```python
from build123d import *

# Parameters (mm, degrees)
SKETCH1_R            = 2.75
BOSS_EXTRUDE1_DEPTH  = 3
M3_CLEARANCE_HOLE1_D = 3.4
FILLET2_R            = 10


with BuildPart() as part:
    # Sketch1 → Boss-Extrude1 (new, symmetric)
    with BuildSketch(Plane(origin=(0, 0, 0), x_dir=(1, 0, 0), z_dir=(0, 1, 0))):
        with BuildLine():
            Line((-58.614111744, 67.959966353), (-53.914904373, 62.511483636))
            ThreePointArc((-53.914904373, 62.511483636), (-82.55, 0), (-53.914904373, -62.511483636))
            Line((-53.914904373, -62.511483636), (-58.614111744, -67.959966353))
            ThreePointArc((-58.614111744, -67.959966353), (-60.384815089, -73.721869234), (-57.34308106, -78.925980035))
            ThreePointArc((-57.34308106, -78.925980035), (-42.766558206, -87.684438581), (-26.890595122, -93.77864983))
            ThreePointArc((-26.890595122, -93.77864983), (-20.917021387, -92.971598421), (-17.46673379, -88.028883515))
            Line((-17.46673379, -88.028883515), (-16.066391761, -80.971436666))
            ThreePointArc((-16.066391761, -80.971436666), (0, -82.55), (16.066391761, -80.971436666))
            Line((16.066391761, -80.971436666), (17.46673379, -88.028883515))
            ThreePointArc((17.46673379, -88.028883515), (20.917021387, -92.971598421), (26.890595122, -93.77864983))
            ThreePointArc((26.890595122, -93.77864983), (42.766558206, -87.684438581), (57.34308106, -78.925980035))
            ThreePointArc((57.34308106, -78.925980035), (60.384815089, -73.721869234), (58.614111744, -67.959966353))
            Line((58.614111744, -67.959966353), (53.914904373, -62.511483636))
            ThreePointArc((53.914904373, -62.511483636), (82.55, 0), (53.914904373, 62.511483636))
            Line((53.914904373, 62.511483636), (58.614111744, 67.959966353))
            ThreePointArc((58.614111744, 67.959966353), (60.384815089, 73.721869234), (57.34308106, 78.925980035))
            ThreePointArc((57.34308106, 78.925980035), (42.766558206, 87.684438581), (26.890595122, 93.77864983))
            ThreePointArc((26.890595122, 93.77864983), (20.917021387, 92.971598421), (17.46673379, 88.028883515))
            Line((17.46673379, 88.028883515), (16.066391761, 80.971436666))
            ThreePointArc((16.066391761, 80.971436666), (0, 82.55), (-16.066391761, 80.971436666))
            Line((-16.066391761, 80.971436666), (-17.46673379, 88.028883515))
            ThreePointArc((-17.46673379, 88.028883515), (-20.917021387, 92.971598421), (-26.890595122, 93.77864983))
            ThreePointArc((-26.890595122, 93.77864983), (-42.766558206, 87.684438581), (-57.34308106, 78.925980035))
            ThreePointArc((-57.34308106, 78.925980035), (-60.384815089, 73.721869234), (-58.614111744, 67.959966353))
        make_face()
        with Locations(Location((52.934691668, -72.858352577, 0), (0, 0, 270))):
            Circle(SKETCH1_R, mode=Mode.SUBTRACT)
        with Locations(Location((52.934691668, 72.858352577, 0), (0, 0, 90))):
            Circle(SKETCH1_R, mode=Mode.SUBTRACT)
    extrude(amount=BOSS_EXTRUDE1_DEPTH, both=True)

    # M3 Clearance Hole1 (through all)
    with Locations(Plane(origin=(0, 3, 0), x_dir=(1, 0, 0), z_dir=(0, 1, 0))):
        with Locations((0, 79.5), (46.728927557, 64.316851053), (75.608993045, 24.566851053), (75.608993045, -24.566851053), (46.728927557, -64.316851053), (0, -79.5), (-46.728927557, -64.316851053), (-75.608993045, -24.566851053), (-75.608993045, 24.566851053), (-46.728927557, 64.316851053)):
            Hole(M3_CLEARANCE_HOLE1_D / 2)

    # Fillet2
    fillet2_edges = [part.edges().sort_by_distance(p)[0] for p in [
        (-53.914904373, 0, 62.511483636),
        (-53.914904373, 0, -62.511483636),
        (-16.066391761, 0, 80.971436666),
        (53.914904373, 0, 62.511483636),
        (53.914904373, 0, -62.511483636),
        (16.066391761, 0, -80.971436666),
        (-16.066391761, 0, -80.971436666),
    ]]
    fillet(fillet2_edges, radius=FILLET2_R)


solid = part.part
```
Source: CAD feature listing. Evaluate the final solid. Frame: model axes, mm. Give positions to 0.01 mm unless a question says otherwise; leave off trailing zeros. Write each loop counter-clockwise with the first axis right and the second up, starting at its lowest first coordinate (ties: lowest second). Pieces come first, ordered by that corner, then holes.
1. Section query C-C (x = -40). Return the cut outline in (y, z), then the cut area to 3 significant figures.
2. Section query A-A (y = 1). Count the separate pieces of the cut face and the enclosed holes in it, then the cut area to 3 significant figures.
3. First-contact query: pin 1 (3 mm diameter, centred on y = 1.5, z = -66, fed in from +X); pin 2 (3 mm diameter, centred on x = 11, y = 2, fed in from -Z). Flat tips, straight axial feed; report the tip coordinate or a pass-through.
4. Pull-direction query (X, two-part tool) for faces 1 (the face through (0.1, 0.04, -82.55)), 2 (the face through (-42.98, 0.04, 87.58)), 3 (the face through (-1, -3, -1)); classes: +X half, -X half, draft (parallel to the pull), parting line (faces both ways), or undercut.
5. Section query B-B (z = -32). Return the cut outline in (x, y), then the cut area to 3 significant figures.
6. Material intervals for line 1 along Z through (x, y) = (0, -0.5); line 2 along Z through (x, y) = (-74.5, -2.25); line 3 along X through (y, z) = (1, 63.5), sorted ascending.
Output values:
1. outline: (-3, -88.98) - (3, -88.98) - (3, 88.98) - (-3, 88.98) - close
1. area: 1,070 mm2
2. separate pieces: 1
2. enclosed holes: 12
2. area: 24,100 mm2
3. pin 1: stops at x = 58.51
3. pin 2: stops at z = -83.13
4. face 1: undercut
4. face 2: -X half
4. face 3: draft
5. outline: (-76.1, -3) - (76.1, -3) - (76.1, 3) - (-76.1, 3) - close
5. area: 913 mm2
6. line 1: z = -82.55 to -81.2, -77.8 to 77.8, 81.2 to 82.55
6. line 2: z = -35.56 to -25.86, -23.28 to 23.28, 25.86 to 35.56
6. line 3: x = -57.57 to -48.22, -45.24 to 45.24, 48.22 to 57.57
